The model under review builds one solid part; all positions refer to its coordinate system, in mm. A direction names the side the tool comes from. Give positions to 0.01 mm unless a question says otherwise; leave off trailing zeros. Loops run counter-clockwise (first coordinate to the right, second up) from the corner with the lowest first, then second, coordinate; pieces in that order, holes last. Notation, with made-up numbers: M 74,44.25 L 117,44.25 A20 ccw 117,72.25 Z; hole C 3,6 d7. An arc over 180 degrees is marked long. Put each result on its own line as item: value. Start each with the question number.
```python
from build123d import *

# Parameters (mm, degrees)
BOSS_EXTRUDE1_DEPTH = 8.1
BOSS_EXTRUDE2_DEPTH = 12.5
FILLET1_R           = 0.5
FILLET2_R           = 0.5
FILLET4_R           = 0.5
CHAMFER2_SIZE       = 1


with BuildPart() as part:
    # Sketch8 → Boss-Extrude1 (new body)
    with BuildSketch(Plane(origin=(-2.232753674, 0, 0.665681661), x_dir=(-1, 0, 0), z_dir=(0, -1, 0))):
        Polygon((-24.744344877, -18.877779499), (-23.219344877, -18.877779499), (-23.219344877, -21.527779499), (-24.744344877, -21.527779499), (-24.744344877, -23.052779499), (-27.394344877, -23.052779499), (-27.394344877, -21.527779499), (-28.919344877, -21.527779499), (-28.919344877, -18.877779499), (-27.394344877, -18.877779499), (-27.394344877, -17.352779499), (-24.744344877, -17.352779499), align=None)
        Polygon((-26.694344877, -20.827779499), (-26.694344877, -22.352779499), (-25.444344877, -22.352779499), (-25.444344877, -20.827779499), (-23.919344877, -20.827779499), (-23.919344877, -19.577779499), (-25.444344877, -19.577779499), (-25.444344877, -18.052779499), (-26.694344877, -18.052779499), (-26.694344877, -19.577779499), (-28.219344877, -19.577779499), (-28.219344877, -20.827779499), align=None, mode=Mode.SUBTRACT)
    extrude(amount=BOSS_EXTRUDE1_DEPTH)

    # Sketch9 → Boss-Extrude2 (add)
    with BuildSketch(Plane(origin=(0, 0, 0), x_dir=(-1, 0, 0), z_dir=(0, 1, 0))):
        with BuildLine():
            Line((-20.086591203, 22.61846116), (-20.086591203, 19.11846116))
            ThreePointArc((-20.086591203, 19.11846116), (-23.836591203, 15.36846116), (-27.586591203, 19.11846116))
            Line((-27.586591203, 19.11846116), (-27.586591203, 22.61846116))
            ThreePointArc((-27.586591203, 22.61846116), (-23.836591203, 26.36846116), (-20.086591203, 22.61846116))
        make_face()
    extrude(amount=BOSS_EXTRUDE2_DEPTH)

    # Fillet1
    fillet1_edges = [part.edges().sort_by_distance(p)[0] for p in [
        (22.511591203, -4.05, 19.54346116),
        (20.986591203, -4.05, 19.54346116),
        (20.986591203, -4.05, 22.19346116),
        (22.511591203, -4.05, 22.19346116),
        (22.511591203, -4.05, 23.71846116),
        (25.161591203, -4.05, 23.71846116),
        (25.161591203, -4.05, 22.19346116),
        (26.686591203, -4.05, 22.19346116),
        (26.686591203, -4.05, 19.54346116),
        (25.161591203, -4.05, 19.54346116),
        (25.161591203, -4.05, 18.01846116),
        (22.511591203, -4.05, 18.01846116),
    ]]
    fillet(fillet1_edges, radius=FILLET1_R)

    # Fillet2
    fillet2_edges = [part.edges().sort_by_distance(p)[0] for p in [
        (21.749091203, 0, 19.54346116),
        (20.986591203, 0, 20.86846116),
        (21.749091203, 0, 22.19346116),
        (22.511591203, 0, 22.95596116),
        (23.836591203, 0, 23.71846116),
        (25.161591203, 0, 22.95596116),
        (25.924091203, 0, 22.19346116),
        (26.686591203, 0, 20.86846116),
        (25.924091203, 0, 19.54346116),
        (25.161591203, 0, 18.78096116),
        (23.836591203, 0, 18.01846116),
        (25.308037813, 0, 19.39701455),
        (25.308037813, 0, 22.339907769),
        (22.365144594, 0, 22.339907769),
        (22.365144594, 0, 19.39701455),
        (21.133037813, 0, 19.689907769),
        (21.133037813, 0, 22.04701455),
        (22.658037813, 0, 23.57201455),
        (25.015144594, 0, 23.57201455),
        (26.540144594, 0, 22.04701455),
        (26.540144594, 0, 19.689907769),
        (22.658037813, 0, 18.164907769),
        (25.015144594, 0, 18.164907769),
        (22.511591203, 0, 18.78096116),
    ]]
    fillet(fillet2_edges, radius=FILLET2_R)

    # Fillet4
    fillet4_edges = [part.edges().sort_by_distance(p)[0] for p in [
        (21.749091203, -8.1, 19.54346116),
        (20.986591203, -8.1, 20.86846116),
        (23.836591203, -8.1, 18.01846116),
        (25.161591203, -8.1, 18.78096116),
        (25.924091203, -8.1, 19.54346116),
        (26.686591203, -8.1, 20.86846116),
        (25.924091203, -8.1, 22.19346116),
        (25.161591203, -8.1, 22.95596116),
        (23.836591203, -8.1, 23.71846116),
        (22.511591203, -8.1, 22.95596116),
        (21.749091203, -8.1, 22.19346116),
        (25.015144594, -8.1, 18.164907769),
        (22.658037813, -8.1, 18.164907769),
        (26.540144594, -8.1, 19.689907769),
        (26.540144594, -8.1, 22.04701455),
        (25.015144594, -8.1, 23.57201455),
        (22.658037813, -8.1, 23.57201455),
        (21.133037813, -8.1, 22.04701455),
        (21.133037813, -8.1, 19.689907769),
        (22.365144594, -8.1, 19.39701455),
        (22.365144594, -8.1, 22.339907769),
        (25.308037813, -8.1, 22.339907769),
        (25.308037813, -8.1, 19.39701455),
        (22.511591203, -8.1, 18.78096116),
    ]]
    fillet(fillet4_edges, radius=FILLET4_R)

    # Chamfer2
    chamfer2_edges = [part.edges().sort_by_distance(p)[0] for p in [
        (23.836591203, 12.5, 26.36846116),
        (27.586591203, 12.5, 20.86846116),
        (23.836591203, 12.5, 15.36846116),
        (20.086591203, 12.5, 20.86846116),
    ]]
    chamfer(chamfer2_edges, length=CHAMFER2_SIZE)


solid = part.part
```
Item 1: Tool access review of faces 4 (the flat face through (20.987, -4, 21)), 5 (the flat face through (23.212, -4, 19)), 6 (the flat face through (24, -4, 23.718)), 7 (the flat face through (20.594, 12.007, 20.893)), 8 (the conical face through (23.77, 12.34, 16.21)): name each direction out of +Z, -Z, +X, -X, +Y, -Y from which nothing blocks a thin tool from reaching the whole face with its end or side.
Item 2: To check wall thickness, follow L1, parallel to Z at x = 23.5, y = -6; L2, parallel to X at y = -2.5, z = 21; L3, parallel to X at y = -6.25, z = 19.75. State the ranges of each line that lie inside material, in increasing order. Write a range as [from, to].
Item 3: Clearance check with flat-ended pins moving along their axes: pin 1 Ø1.7 at (y, z) = (-5, 22.5) entering from -X; pin 2 Ø3 at (x, y) = (26, 5) entering from -Z; pin 3 Ø1.2 at (x, y) = (25, -5.5) entering from +Z. State where each tip first meets the part, or that it passes through.
Item 4: Consider section A-A, the plane z = 21.25. Write out the cut boundary in (x, y).
Item 5: Draft analysis for pull direction Z (two halves, no side actions). For faces 1 (the flat face through (25, -8.1, 20)), 2 (the flat face through (24, -4, 18.018)), 3 (the flat face through (22, -4, 20.243)), state which applies: +Z half, -Z half, draft (parallel to the pull), parting line (faces both ways), or undercut.
Item 6: Consider section B-B, the plane y = 10.75. Write out the cut boundary in (x, z), plus the area to 3 significant figures.
Report:
1. face 4: +Z, -Z, -X, -Y
1. face 5: -Y
1. face 6: +Z, +X, -X, -Y
1. face 7: +Z, -Z, -X, +Y
1. face 8: -Z, +Y
2. L1: [18.02, 18.72], [23.02, 23.72]
2. L2: [20.99, 21.69], [25.99, 26.69]
2. L3: [21.08, 23.21], [24.46, 26.59]
3. pin 1: x = 20.99
3. pin 2: z = 15.43
3. pin 3: z = 23.72
4. outline: M 20.09,0 L 20.49,0 A0.5 cw 20.99,-0.5 L 20.99,-7.6 A0.5 ccw 21.49,-8.1 L 21.69,-8.1 L 21.69,0 L 25.99,0 L 25.99,-8.1 L 26.19,-8.1 A0.5 ccw 26.69,-7.6 L 26.69,-0.5 A0.5 cw 27.19,0 L 27.59,0 L 27.59,11.5 L 26.59,12.5 L 21.09,12.5 L 20.09,11.5 Z
5. face 1: draft
5. face 2: -Z half
5. face 3: undercut
6. outline: M 20.09,19.12 A3.75 ccw 27.59,19.12 L 27.59,22.62 A3.75 ccw 20.09,22.62 Z
6. area: 70.4 mm²
